Autodesk Inventor part; units mm, degrees
ref_plane "YZ Plane" through (0, 0, 0) normal (1, 0, 0) x (0, 1, 0)
ref_plane "XZ Plane" through (0, 0, 0) normal (0, 1, 0) x (-1, 0, 0)
ref_plane "XY Plane" through (0, 0, 0) normal (0, 0, 1) x (1, 0, 0)
sketch "Sketch1" plane through (0, 0, 0) normal (0, 0, 1) x (1, 0, 0)
  line L0 (0, 21.9424) -> (0, -17.6259)
  line L1 (4, 26.2687) -> (4, 2.2687)
  line L2 (4, 2.2687) -> (7, 2.2687)
  line L3 (7, 2.2687) -> (7.5, 2.7687)
  line L4 (7.5, 2.7687) -> (7.5, 6.2687)
  line L5 (7.5, 6.2687) -> (7, 6.2687)
  line L6 (7, 6.2687) -> (7, 7.2687)
  line L7 (7, 7.2687) -> (7.5, 7.2687)
  line L8 (7.5, 7.2687) -> (7.5, 21.2687)
  line L9 (7.5, 21.2687) -> (7, 21.2687)
  line L10 (7, 21.2687) -> (7, 22.2687)
  line L11 (7, 22.2687) -> (7.5, 22.2687)
  line L12 (7.5, 22.2687) -> (7.5, 25.7687)
  line L13 (7.5, 25.7687) -> (7, 26.2687)
  line L14 (7, 26.2687) -> (4, 26.2687)
  dimension "d1" = 1
  dimension "d2" = 1
  dimension "d3" = 0.5
  dimension "d4" = 0.5
  dimension "d5" = 0.5
  dimension "d6" = 0.5
  dimension "d7" = 24
  dimension "d8" = 8
  dimension "d9" = 15
  dimension "d10" = 4
  dimension "d11" = 4
  dimension "d12" = 0.5
revolve "Revolution1" add sketch "Sketch1" angle 360 about axis through (0, 21.9424, 0) along (0, -1, 0)
properties part number "lm8uu"
Source: CAD feature listing. Evaluate the final solid. Frame: model axes, mm. A direction names the side the tool comes from. Round coordinates to 2 decimals unless told otherwise and drop trailing zeros. Write each loop counter-clockwise with the first axis right and the second up, starting at its lowest first coordinate (ties: lowest second). Pieces come first, ordered by that corner, then holes. Notation, with made-up numbers: M 42,50 L 75,50 A10 cw 75,58 Z; hole C -37,-35.75 d4. An arc over 180 degrees is marked long. Use CSV: the item, a comma, the result in double quotes. Start each with the question number.
Q1. First-contact query: P1, Ø3, axis at x = -4.5, y = 22, coming from the +Z side; P2, Ø4, axis at y = 17, z = 5, coming from the +X side; P3, Ø6, axis at x = -4.5, y = 13.5, coming from the -Z side. Flat tips, straight axial feed; report the tip coordinate or a pass-through.
Q2. Cut plane A-A on x = 0. Output: boundary loops of the cut face in (y, z), plus the area to 4 significant figures.
Q3. Line query: line 1 (Z direction, x = 0, y = 17.75); line 2 (X direction, y = 23.25, z = 1.5); line 3 (Z direction, x = 3, y = 8.5). Output: solid intervals per line, ascending. Write a range as from..to.
Q4. Cut plane B-B on z = 0. Output: boundary loops of the cut face in (x, y), plus the area to 4 significant figures.
Q5. Access query for faces 4 (the face through (7, 22.269, 2)), 5 (the face through (-7.493, 4.543, -0.33)). Directions: +Z, -Z, +X, -X, +Y, -Y. A direction counts if a zero-diameter tool reaches every point of the face in a straight line with its end or side. Return the directions, or none.
Q6. Pull-direction query (Y, two-part tool) for faces 1 (the face through (-0.867, 14.101, -3.905)), 2 (the face through (3, 26.269, -3)), 3 (the face through (7, 6.269, 2)); classes: +Y half, -Y half, draft (parallel to the pull), parting line (faces both ways), or undercut.
Q7. Cut plane C-C on y = 13. Output: boundary loops of the cut face in (x, z), plus the area to 3 significant figures.
Results found:
1,P1,"z = 6.86"
1,P2,"x = 6.87"
1,P3,"z = -7.35"
2,outline,"M 2.27,-7 L 2.77,-7.5 L 6.27,-7.5 L 6.27,-7 L 7.27,-7 L 7.27,-7.5 L 21.27,-7.5 L 21.27,-7 L 22.27,-7 L 22.27,-7.5 L 25.77,-7.5 L 26.27,-7 L 26.27,-4 L 2.27,-4 Z; M 2.27,4 L 26.27,4 L 26.27,7 L 25.77,7.5 L 22.27,7.5 L 22.27,7 L 21.27,7 L 21.27,7.5 L 7.27,7.5 L 7.27,7 L 6.27,7 L 6.27,7.5 L 2.77,7.5 L 2.27,7 Z"
2,area,"165.5 mm^2"
3,line 1,"-7.5..-4, 4..7.5"
3,line 2,"-7.35..-3.71, 3.71..7.35"
3,line 3,"-6.87..-2.65, 2.65..6.87"
4,outline,"M -7.5,2.77 L -7,2.27 L -4,2.27 L -4,26.27 L -7,26.27 L -7.5,25.77 L -7.5,22.27 L -7,22.27 L -7,21.27 L -7.5,21.27 L -7.5,7.27 L -7,7.27 L -7,6.27 L -7.5,6.27 Z; M 4,2.27 L 7,2.27 L 7.5,2.77 L 7.5,6.27 L 7,6.27 L 7,7.27 L 7.5,7.27 L 7.5,21.27 L 7,21.27 L 7,22.27 L 7.5,22.27 L 7.5,25.77 L 7,26.27 L 4,26.27 Z"
4,area,"165.5 mm^2"
5,face 4,"none"
5,face 5,"+Y, -Y"
6,face 1,"draft"
6,face 2,"+Y half"
6,face 3,"undercut"
7,outline,"C 0,0 d15; hole C 0,0 d8"
7,area,"126 mm^2"
